from build123d import *

# Parameters (mm, degrees)
SKETCH1_W                = 10.2
SKETCH1_H                = 5.2
BOSS_EXTRUDE1_DEPTH      = 7.05
CHAMFER1_SIZE            = 1.5
BOSS_EXTRUDE2_DEPTH      = 10.05
BOSS_EXTRUDE2_DEPTH_BACK = 10.05
SKETCH2_R                = 0.875


with BuildPart() as part:
    # Sketch1 → Boss-Extrude1 (new, symmetric)
    with BuildSketch(Plane(origin=(0, 0, 0), x_dir=(1, 0, 0), z_dir=(0, 1, 0))):
        Rectangle(SKETCH1_W, SKETCH1_H)
    extrude(amount=BOSS_EXTRUDE1_DEPTH, both=True)

    # Chamfer1
    chamfer1_edges = [part.edges().sort_by_distance(p)[0] for p in [
        (5.1, 0, 2.6),
        (5.1, 0, -2.6),
    ]]
    chamfer(chamfer1_edges, length=CHAMFER1_SIZE)

    # Sketch2 → Boss-Extrude2 (add, two sides: drawn at the far end of the back side and taken through both)
    with BuildSketch(Plane(origin=(0, 0, 0), x_dir=(1, 0, 0), z_dir=(0, 1, 0)).offset(-BOSS_EXTRUDE2_DEPTH_BACK)):
        with Locations(Location((-2.5, 0, 0), (0, 0, 90))):
            Circle(SKETCH2_R)
        with Locations(Location((2.5, 0, 0), (0, 0, 90))):
            Circle(SKETCH2_R)
    extrude(amount=BOSS_EXTRUDE2_DEPTH + BOSS_EXTRUDE2_DEPTH_BACK)


solid = part.part
Source: CAD feature listing. Evaluate the final solid. Frame: model axes, mm. A direction names the side the tool comes from. Round coordinates to 2 decimals unless told otherwise and drop trailing zeros. Loops run counter-clockwise (first coordinate to the right, second up) from the corner with the lowest first, then second, coordinate; pieces in that order, holes last.
Q1. Section D-D, the plane y = -8.5. Return loops of the section in (x, z) (3 decimals).
Q2. Section C-C, the plane y = -3. Return loops of the section in (x, z), plus the area to 3 significant figures.
Q3. Section B-B, the plane z = 0. Return loops of the section in (x, y) (3 decimals).
Q4. Section A-A, the plane x = -2.5. Return loops of the section in (y, z) (3 decimals).
Q5. Mould query, pull axis X, two halves, no side actions, for faces 1 (the face through (-1.646, 8.529, 0.19)), 2 (the face through (3.354, 8.529, 0.19)), 3 (the face through (-5.1, 0, 0)), 4 (the face through (-3, 10.05, 0)). Classes: pulls with the +X half, pulls with the -X half, needs draft (parallel to the pull), parting line crosses it, or undercut.
Q6. Ray query, line 1 (X direction, y = -7.5, z = 0) (3 decimals); line 2 (Y direction, x = 1.75, z = 1.45); line 3 (X direction, y = -8, z = -0.7) (3 decimals). Return the intervals inside material, ascending.
Q7. Access query for faces 5 (the face through (-1, 0, -2.6)), 6 (the face through (3.354, -8.571, 0.19)), 7 (the face through (0, 7.05, 0)). Directions: +Z, -Z, +X, -X, +Y, -Y. A direction counts if a zero-diameter tool reaches every point of the face in a straight line with its end or side. Return the directions, or none.
Q8. First-contact query: P1, Ø1.6, axis at x = 0.5, z = -1, coming from the +Y side. Flat tip, straight axial feed; report the tip coordinate or a pass-through.
Solutions:
1. outline: circle Ø1.75 at (-2.5, 0); circle Ø1.75 at (2.5, 0)
2. outline: (-5.1, -2.6) - (3.6, -2.6) - (5.1, -1.1) - (5.1, 1.1) - (3.6, 2.6) - (-5.1, 2.6) - close
2. area: 50.8 mm2
3. outline: (-5.1, -7.05) - (-3.375, -7.05) - (-3.375, -10.05) - (-1.625, -10.05) - (-1.625, -7.05) - (1.625, -7.05) - (1.625, -10.05) - (3.375, -10.05) - (3.375, -7.05) - (5.1, -7.05) - (5.1, 7.05) - (3.375, 7.05) - (3.375, 10.05) - (1.625, 10.05) - (1.625, 7.05) - (-1.625, 7.05) - (-1.625, 10.05) - (-3.375, 10.05) - (-3.375, 7.05) - (-5.1, 7.05) - close
4. outline: (-10.05, -0.875) - (-7.05, -0.875) - (-7.05, -2.6) - (7.05, -2.6) - (7.05, -0.875) - (10.05, -0.875) - (10.05, 0.875) - (7.05, 0.875) - (7.05, 2.6) - (-7.05, 2.6) - (-7.05, 0.875) - (-10.05, 0.875) - close
5. face 1: undercut
5. face 2: undercut
5. face 3: pulls with the -X half
5. face 4: needs draft
6. line 1: x = -3.375 to -1.625, 1.625 to 3.375
6. line 2: y = -7.05 to 7.05
6. line 3: x = -3.025 to -1.975, 1.975 to 3.025
7. face 5: -Z, +X, -X, +Y, -Y
7. face 6: -Y
7. face 7: +Y
8. P1: stops at y = 7.05
